For this review, take the finished solid that the model builds, in its own axes (mm). A direction names the side the tool comes from. Coordinates: 2 decimals unless noted, no trailing zeros. Write each loop counter-clockwise with the first axis right and the second up, starting at its lowest first coordinate (ties: lowest second). Pieces come first, ordered by that corner, then holes. Notation, with made-up numbers: (85, 68) - (141, 68) arc R8 cw to (141, 77) - close; hole circle Ø6 at (82.5, 53.25). An arc over 180 degrees is marked (long way). Use one line per item in the form item = value. Start each with the question number.
1) Insertion check: P1, Ø9.5, axis at x = 11.5, y = 64, coming from the -Z side (3 decimals). The pin has a flat end and moves straight along its axis. Give the tip position at first contact, or say it passes through.
2) We need section A-A (z = 3). Give the boundary of the cut face in (x, y) (3 decimals), plus the area to 3 significant figures.
3) For L1, parallel to Y at x = -34, z = 9; L2, parallel to Z at x = -240.5, y = 67 (3 decimals); L3, parallel to X at y = 94, z = 7.5, list the stretches that pass through material, from the lowest coordinate up. Write a range as from..to.
4) Tool access review of faces 1 (the flat face through (4, 50.8, 5)), 2 (the flat face through (-301.625, 42, 9)): name each direction out of +Z, -Z, +X, -X, +Y, -Y from which nothing blocks a thin tool from reaching the whole face with its end or side.
5) Mouldability with a two-part tool opening along Y and no side actions: class faces 3 (the cylindrical face through (296.66, 96.89, 9.66)), 4 (the flat face through (-4, 26, 0)), 5 (the flat face through (4, 60, 9.525)) as pulls with the +Y half, pulls with the -Y half, needs draft (parallel to the pull), parting line crosses it, or undercut.
6) We need section B-B (x = 161.5). Give the boundary of the cut face in (y, z) (3 decimals).
```python
from build123d import *

# Parameters (mm, degrees)
SKETCH1_W           = 603.25
SKETCH1_H           = 101.6
BOSS_EXTRUDE1_DEPTH = 19.05
SKETCH2_W           = 9.525
SKETCH2_H           = 19.05
CUT_EXTRUDE1_DEPTH  = 613.042502609
FILLET1_R           = 16.51


with BuildPart() as part:
    # Sketch1 → Boss-Extrude1 (new body)
    with BuildSketch(Plane.XY):
        with Locations((0, 50.8)):
            Rectangle(SKETCH1_W, SKETCH1_H)
    extrude(amount=BOSS_EXTRUDE1_DEPTH)

    # Sketch2 → Cut-Extrude1 (cut, through all)
    with BuildSketch(Plane(origin=(301.625, 0, 0), x_dir=(0, 0, -1), z_dir=(1, 0, 0))):
        with Locations((-4.7625, 60.325)):
            Rectangle(SKETCH2_W, SKETCH2_H)
    extrude(amount=-CUT_EXTRUDE1_DEPTH, mode=Mode.SUBTRACT)

    # Fillet1
    fillet1_edges = [part.edges().sort_by_distance(p)[0] for p in [
        (301.625, 101.6, 9.525),
        (-301.625, 101.6, 9.525),
    ]]
    fillet(fillet1_edges, radius=FILLET1_R)


solid = part.part
```
Determined:
q1.P1 = 9.525
q2.outline = (-301.625, 0) - (301.625, 0) - (301.625, 50.8) - (-301.625, 50.8) - close; (-301.625, 69.85) - (301.625, 69.85) - (301.625, 85.09) arc R16.51 ccw to (285.115, 101.6) - (-285.115, 101.6) arc R16.51 ccw to (-301.625, 85.09) - close
q2.area = 49,700 mm²
q3.L1 = 0..50.8, 69.85..101.6
q3.L2 = 9.525..19.05
q3.L3 = -299.01..299.01
q4.face_1 = -Z, +X, -X
q4.face_2 = +Z, -Z, -X, +Y, -Y
q5.face_3 = pulls with the +Y half
q5.face_4 = needs draft
q5.face_5 = undercut
q6.outline = (0, 0) - (50.8, 0) - (50.8, 9.525) - (69.85, 9.525) - (69.85, 0) - (101.6, 0) - (101.6, 19.05) - (0, 19.05) - close
